```python
from build123d import *

# Parameters (mm, degrees)
BOSS_EXTRUDE1_DEPTH = 3
SKETCH2_R           = 3.2
CUT_EXTRUDE1_DEPTH  = 3
SKETCH5_R           = 2
CUT_EXTRUDE2_DEPTH  = 3
SKETCH10_R          = 2
CUT_EXTRUDE4_DEPTH  = 3


with BuildPart() as part:
    # Sketch1 → Boss-Extrude1 (new body)
    with BuildSketch(Plane.XY):
        with BuildLine():
            Line((0, 5), (330, 5))
            ThreePointArc((330, 5), (335, 0), (330, -5))
            Line((330, -5), (0, -5))
            ThreePointArc((0, -5), (-5, 0), (0, 5))
        make_face()
    extrude(amount=BOSS_EXTRUDE1_DEPTH)

    # Sketch2 → Cut-Extrude1 (cut)
    with BuildSketch(Plane.XY.offset(3)):
        with Locations((323, 0)):
            Circle(SKETCH2_R)
    extrude(amount=-CUT_EXTRUDE1_DEPTH, mode=Mode.SUBTRACT)

    # Sketch5 → Cut-Extrude2 (cut)
    with BuildSketch(Plane.XY.offset(3)):
        with Locations((190, 0)):
            Circle(SKETCH5_R)
    extrude(amount=-CUT_EXTRUDE2_DEPTH, mode=Mode.SUBTRACT)

    # Sketch10 → Cut-Extrude4 (cut)
    with BuildSketch(Plane.XY.offset(3)):
        Circle(SKETCH10_R)
    extrude(amount=-CUT_EXTRUDE4_DEPTH, mode=Mode.SUBTRACT)


solid = part.part
```
The listing builds one solid part. Answer for the finished solid, in the listing's coordinates (mm). Coordinates: 2 decimals unless noted, no trailing zeros. Write each loop counter-clockwise with the first axis right and the second up, starting at its lowest first coordinate (ties: lowest second). Pieces come first, ordered by that corner, then holes. Notation, with made-up numbers: (88.5, 76.5) - (96.5, 76.5) arc R19 ccw to (96.5, 89.5) - close; hole circle Ø5 at (85, 11). An arc over 180 degrees is marked (long way). Return JSON: item names as keys, results as strings. Group by question number.
1. A cutting plane is placed at B-B, the plane x = 323. Determine the outline of the cut face in (y, z).
2. Straight lines are drawn through the part: L1, parallel to X at y = 0.5, z = 0.15; L2, parallel to X at y = 1.25, z = 1.9; L3, parallel to Y at x = 190, z = 1.4. For each, find the intervals that lie inside material, in ascending order.
3. Determine the mould class of faces 1 (the flat face through (167, 0, 0)), 2 (the cylindrical face through (325.956, -1.226, 1.521)) for opening direction X: released by +X, released by -X, zero draft, split by the parting line, or undercut.
4. Given pin 1 (3 mm diameter, centred on x = 0, y = 0, fed in from +Z); pin 2 (1.5 mm diameter, centred on y = -1, z = 1, fed in from -X), each flat-ended and moving along its own axis, determine where each tip first touches the part or whether it passes through.
5. A cutting plane is placed at A-A, the plane y = 0. Determine the outline of the cut face in (x, z).
6. A cutting plane is placed at C-C, the plane z = 0.75. Determine the outline of the cut face in (x, y).
Ans:
{
 "1": {"outline": "(-5, 0) - (-3.2, 0) - (-3.2, 3) - (-5, 3) - close; (3.2, 0) - (5, 0) - (5, 3) - (3.2, 3) - close"},
 "2": {"L1": "-4.97 to -1.94, 1.94 to 188.06, 191.94 to 319.84, 326.16 to 334.97", "L2": "-4.84 to -1.56, 1.56 to 188.44, 191.56 to 320.05, 325.95 to 334.84", "L3": "-5 to -2, 2 to 5"},
 "3": {"face 1": "zero draft", "face 2": "undercut"},
 "4": {"pin 1": "through", "pin 2": "x = -4.99"},
 "5": {"outline": "(-5, 0) - (-2, 0) - (-2, 3) - (-5, 3) - close; (2, 0) - (188, 0) - (188, 3) - (2, 3) - close; (192, 0) - (319.8, 0) - (319.8, 3) - (192, 3) - close; (326.2, 0) - (335, 0) - (335, 3) - (326.2, 3) - close"},
 "6": {"outline": "(0, -5) - (330, -5) arc R5 ccw to (330, 5) - (0, 5) arc R5 ccw to start; hole circle Ø4 at (0, 0); hole circle Ø4 at (190, 0); hole circle Ø6.4 at (323, 0)"}
}
